Can you work these out from the drawing? Everything is in mm from the part's minimum corner. Give positions to 0.01 mm unless a question says otherwise; leave off trailing zeros. Write each loop counter-clockwise with the first axis right and the second up, starting at its lowest first coordinate (ties: lowest second). Pieces come first, ordered by that corner, then holes. Notation, with made-up numbers: M 12.25,19.5 L 23.25,19.5 A26 ccw 23.25,57.5 Z; hole C 3,87 d4. An arc over 180 degrees is marked long. One line per item, written item: value.
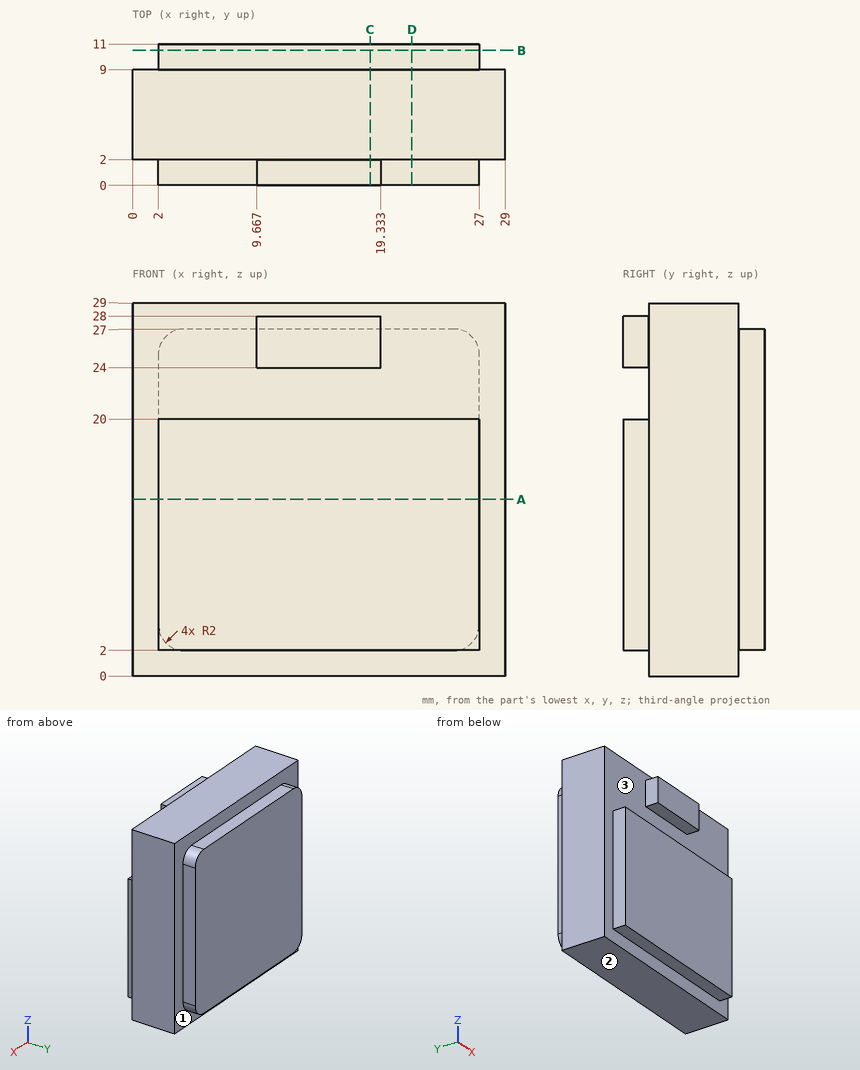
1) If we section it at C-C, the plane x = 18.5: Write out the boundary of the cut face in (y, z), then the cut area to 3 significant figures.
Outcome:
outline: M 0,2 L 2,2 L 2,0 L 9,0 L 9,2 L 11,2 L 11,27 L 9,27 L 9,29 L 2,29 L 2,28 L 0,28 L 0,24 L 2,24 L 2,20 L 0,20 Z
area: 297 mm^2
2) We'd pull the mould along Z, two halves only. Please class the marked faces 1, 2 and 3: pulls with the +Z half, pulls with the -Z half, needs draft (parallel to the pull), parting line crosses it, or undercut.
Outcome:
face 1: needs draft
face 2: pulls with the -Z half
face 3: undercut
3) If we section it at A-A, the plane z = 13.75: Write out the boundary of the cut face in (x, y).
Outcome:
outline: M 0,2 L 2,2 L 2,0 L 27,0 L 27,2 L 29,2 L 29,9 L 27,9 L 27,11 L 2,11 L 2,9 L 0,9 Z
4) If we section it at D-D, the plane x = 21.75: Write out the boundary of the cut face in (y, z), then the cut area to 3 significant figures.
Outcome:
outline: M 0,2 L 2,2 L 2,0 L 9,0 L 9,2 L 11,2 L 11,27 L 9,27 L 9,29 L 2,29 L 2,20 L 0,20 Z
area: 289 mm^2
5) Please list where these lines run through material, in increasing order: L1, parallel to X at y = 1.25, z = 2.75; L2, parallel to Y at x = 24.75, z = 22.5; L3, parallel to Y at x = 27.75, z = 10.75. Write a range as from..to.
Outcome:
L1: x = 2..27
L2: y = 2..11
L3: y = 2..9
6) I'm going to push flat-ended pins straight in: pin 1 (3 mm diameter, centred on x = 12.5, y = 7.5, fed in from -Z); pin 2 (1 mm diameter, centred on y = 10.5, z = 14.5, fed in from +X); pin 3 (1 mm diameter, centred on x = 13.5, y = 0.5, fed in from -Z); pin 4 (1.6 mm diameter, centred on x = 14, y = 1, fed in from +Z). Where does each tip first touch, or does it pass through?
Outcome:
pin 1: stops at z = 0
pin 2: stops at x = 27
pin 3: stops at z = 2
pin 4: stops at z = 28
7) If we section it at B-B, the plane y = 10.5: Write out the boundary of the cut face in (x, z).
Outcome:
outline: M 2,4 A2 ccw 4,2 L 25,2 A2 ccw 27,4 L 27,25 A2 ccw 25,27 L 4,27 A2 ccw 2,25 Z
